Check sheet for the modelled part. Datum: model origin and axes. Units: mm. A direction names the side the tool comes from. Round coordinates to 2 decimals unless told otherwise and drop trailing zeros. Loops run counter-clockwise (first coordinate to the right, second up) from the corner with the lowest first, then second, coordinate; pieces in that order, holes last. Notation, with made-up numbers: (-3, 27) -> (51, 27) arc R37 ccw to (51, 63) -> close; hole circle Ø4 at (-29, 64). An arc over 180 degrees is marked (long way). One line per item, written item: value. Start each with the question number.
1. Cross-section at D-D on x = 4.5. Record the cut outline in (y, z), then the cut area to 3 significant figures.
2. Set-up check for faces 1 (the face through (-7.6, 27, 0)), 2 (the face through (-12.5, 28, 0)), 3 (the face through (-10, 55, 0)): record each of +Z, -Z, +X, -X, +Y, -Y from which the full face is reachable in a straight line by a thin tool's end or side.
3. Cross-section at B-B on y = 50. Count the separate pieces of the cut face and the enclosed holes in it, then the cut area to 3 significant figures.
4. Cross-section at A-A on y = 16.5. Record the cut outline in (x, z).
5. Material ranges on L1, parallel to X at y = 42.5, z = -10.5; L2, parallel to Y at x = -8.7, z = -10; L3, parallel to Y at x = -7.5, z = 14.5, recorded low to high.
6. Cross-section at C-C on z = -10. Record the cut outline in (x, y).
7. Go/stop test with flat-tipped pins: pin 1 (10 mm diameter, centred on y = 47, z = 2, fed in from -X); pin 2 (9 mm diameter, centred on x = -19.5, z = 2, fed in from +Y); pin 3 (6 mm diameter, centred on y = 32.5, z = -5, fed in from +X). Record where each tip stops, or that it passes through.
8. Release check for a two-part mould opening along X. For faces 4 (the face through (7.45, 28, 0)), 5 (the face through (5, 55, 0)), 6 (the face through (2.55, 27, 0)) record: +X half, -X half, draft (parallel to the pull), parting line (faces both ways), or undercut.
from build123d import *

# Parameters (mm, degrees)
SKETCH1_W             = 4.9
SKETCH1_H             = 40
BOSS_EXTRUDE1_DEPTH   = 55
BOSS_EXTRUDE1_2_DEPTH = 55
SKETCH2_W             = 19.95
SKETCH2_H             = 40
BOSS_EXTRUDE2_DEPTH   = 10
SKETCH3_R             = 2.5
CUT_EXTRUDE1_DEPTH    = 19.95
SKETCH5_W             = 40
SKETCH5_H             = 10
BOSS_EXTRUDE4_DEPTH   = 10
SKETCH6_W             = 40
SKETCH6_H             = 10
BOSS_EXTRUDE5_DEPTH   = 10
FILLET1_R             = 1


with BuildPart() as part:
    # Sketch1 → Boss-Extrude1 (new body)
    with BuildSketch(Plane(origin=(0, 0, 0), x_dir=(1, 0, 0), z_dir=(0, 1, 0))):
        with Locations((-10.05, 0)):
            Rectangle(SKETCH1_W, SKETCH1_H)
    extrude(amount=BOSS_EXTRUDE1_DEPTH)



with BuildPart() as body_2:
    # Sketch1 → Boss-Extrude1 2 (new body)
    with BuildSketch(Plane(origin=(0, 0, 0), x_dir=(1, 0, 0), z_dir=(0, 1, 0))):
        with Locations((5, 0)):
            Rectangle(SKETCH1_W, SKETCH1_H)
    extrude(amount=BOSS_EXTRUDE1_2_DEPTH)


with BuildPart() as part_1:
    add(part.part)

    add(body_2.part)  # Boss-Extrude2 merges body 2
    # Sketch2 → Boss-Extrude2 (add)
    with BuildSketch(Plane.XZ):
        with Locations((-2.525, 0)):
            Rectangle(SKETCH2_W, SKETCH2_H)
    extrude(amount=BOSS_EXTRUDE2_DEPTH)

    # Sketch3 → Cut-Extrude1 (cut)
    with BuildSketch(Plane.ZY.offset(12.5)):
        with Locations((-10, 50)):
            Circle(SKETCH3_R)
        with Locations((10, 50)):
            Circle(SKETCH3_R)
    extrude(amount=-CUT_EXTRUDE1_DEPTH, mode=Mode.SUBTRACT)

    # Sketch5 → Boss-Extrude4 (add)
    with BuildSketch(Plane.ZY.offset(12.5)):
        with Locations((0, -5)):
            Rectangle(SKETCH5_W, SKETCH5_H)
    extrude(amount=BOSS_EXTRUDE4_DEPTH)

    # Sketch6 → Boss-Extrude5 (add)
    with BuildSketch(Plane(origin=(7.45, 0, 0), x_dir=(0, 0, -1), z_dir=(1, 0, 0))):
        with Locations((0, -5)):
            Rectangle(SKETCH6_W, SKETCH6_H)
    extrude(amount=BOSS_EXTRUDE5_DEPTH)

    # Fillet1
    fillet1_edges = [part_1.edges().sort_by_distance(p)[0] for p in [
        (2.55, 27.5, -20),
        (2.55, 27.5, 20),
        (-22.5, -5, -20),
        (-22.5, -5, 20),
        (-12.5, 27.5, -20),
        (7.45, 27.5, -20),
        (7.45, 27.5, 20),
        (-7.6, 27.5, -20),
        (-7.6, 27.5, 20),
        (17.45, -5, 20),
        (-12.5, 27.5, 20),
        (17.45, -5, -20),
    ]]
    fillet(fillet1_edges, radius=FILLET1_R)


solid = part_1.part
Taken from the geometry:
1. outline: (-10, -20) -> (55, -20) -> (55, 20) -> (-10, 20) -> close; hole circle Ø5 at (50, -10); hole circle Ø5 at (50, 10)
1. area: 2,560 mm2
2. face 1: +Z, -Z, +Y
2. face 2: +Z, -Z, -X, +Y
2. face 3: +Z, -Z, +X, -X, +Y
3. separate pieces: 6
3. enclosed holes: 0
3. area: 292 mm2
4. outline: (-12.5, -19) arc R1 ccw to (-11.5, -20) -> (-8.6, -20) arc R1 ccw to (-7.6, -19) -> (-7.6, 19) arc R1 ccw to (-8.6, 20) -> (-11.5, 20) arc R1 ccw to (-12.5, 19) -> close; (2.55, -19) arc R1 ccw to (3.55, -20) -> (6.45, -20) arc R1 ccw to (7.45, -19) -> (7.45, 19) arc R1 ccw to (6.45, 20) -> (3.55, 20) arc R1 ccw to (2.55, 19) -> close
5. L1: x = -12.5 to -7.6, 2.55 to 7.45
5. L2: y = -10 to 47.5, 52.5 to 55
5. L3: y = -10 to 0
6. outline: (-22.5, -10) -> (17.45, -10) -> (17.45, 0) -> (7.45, 0) -> (7.45, 47.5) -> (2.55, 47.5) -> (2.55, 0) -> (-7.6, 0) -> (-7.6, 47.5) -> (-12.5, 47.5) -> (-12.5, 0) -> (-22.5, 0) -> close; (-12.5, 52.5) -> (-7.6, 52.5) -> (-7.6, 55) -> (-12.5, 55) -> close; (2.55, 52.5) -> (7.45, 52.5) -> (7.45, 55) -> (2.55, 55) -> close
7. pin 1: stops at x = -12.5
7. pin 2: stops at y = 0
7. pin 3: stops at x = 7.45
8. face 4: +X half
8. face 5: draft
8. face 6: undercut
